from build123d import *

# Parameters (mm, degrees)
SALIENTE_EXTRUIR1_DEPTH = 1.5
CROQUIS2_R              = 1.6
CORTAR_EXTRUIR1_DEPTH   = 10
CROQUIS3_W              = 12
CROQUIS3_H              = 6
CORTAR_EXTRUIR2_DEPTH   = 10
CROQUIS4_W              = 4
CROQUIS4_H              = 16
CORTAR_EXTRUIR3_DEPTH   = 10
CORTAR_EXTRUIR4_REACH   = 107.991
CROQUIS5_R              = 1.5


with BuildPart() as part:
    # Croquis1 → Saliente-Extruir1 (new, symmetric)
    with BuildSketch(Plane.XY):
        Polygon((-75, -32), (-75, -35), (-45, -35), (-45, -32), (45, -32), (45, -35), (75, -35), (75, -32), (97, -32), (97, -12.5), (100, -12.5), (100, 12.5), (97, 12.5), (97, 32), (75, 32), (75, 35), (45, 35), (45, 32), (-45, 32), (-45, 35), (-75, 35), (-75, 32), (-97, 32), (-97, 12.5), (-100, 12.5), (-100, -12.5), (-97, -12.5), (-97, -32), align=None)
    extrude(amount=SALIENTE_EXTRUIR1_DEPTH, both=True)

    # Croquis2 → Cortar-Extruir1 (cut)
    with BuildSketch(Plane.XY.offset(1.5)):
        with Locations((72.948592978, -19.354512833)):
            Circle(CROQUIS2_R)
        with Locations((88.948592978, -19.354512833)):
            Circle(CROQUIS2_R)
    extrude(amount=-CORTAR_EXTRUIR1_DEPTH, mode=Mode.SUBTRACT)

    # Croquis3 → Cortar-Extruir2 (cut)
    with BuildSketch(Plane.XY.offset(1.5)):
        with Locations((81, -25)):
            Rectangle(CROQUIS3_W, CROQUIS3_H)
    extrude(amount=-CORTAR_EXTRUIR2_DEPTH, mode=Mode.SUBTRACT)

    # Croquis4 → Cortar-Extruir3 (cut)
    with BuildSketch(Plane.XY.offset(1.5)):
        with Locations((66.93, 0)):
            Rectangle(CROQUIS4_W, CROQUIS4_H)
    extrude(amount=-CORTAR_EXTRUIR3_DEPTH, mode=Mode.SUBTRACT)

    # Croquis5 → Cortar-Extruir4 (cut, up to next)
    with BuildSketch(Plane.XY.offset(1.5), mode=Mode.PRIVATE) as cortar_extruir4_sk1:
        with Locations((21.93, 9.75)):
            Circle(CROQUIS5_R)
    cortar_extruir4_tool1 = extrude(cortar_extruir4_sk1.sketch, amount=-CORTAR_EXTRUIR4_REACH, mode=Mode.PRIVATE) & part.part
    # Croquis5 → Cortar-Extruir4 (cut, up to next)
    with BuildSketch(Plane.XY.offset(1.5), mode=Mode.PRIVATE) as cortar_extruir4_sk2:
        with Locations((21.93, -9.75)):
            Circle(CROQUIS5_R)
    cortar_extruir4_tool2 = extrude(cortar_extruir4_sk2.sketch, amount=-CORTAR_EXTRUIR4_REACH, mode=Mode.PRIVATE) & part.part
    # Croquis5 → Cortar-Extruir4 (cut, up to next)
    with BuildSketch(Plane.XY.offset(1.5), mode=Mode.PRIVATE) as cortar_extruir4_sk3:
        with Locations((-46.07, -9.75)):
            Circle(CROQUIS5_R)
    cortar_extruir4_tool3 = extrude(cortar_extruir4_sk3.sketch, amount=-CORTAR_EXTRUIR4_REACH, mode=Mode.PRIVATE) & part.part
    # Croquis5 → Cortar-Extruir4 (cut, up to next)
    with BuildSketch(Plane.XY.offset(1.5), mode=Mode.PRIVATE) as cortar_extruir4_sk4:
        with Locations((-46.07, 9.75)):
            Circle(CROQUIS5_R)
    cortar_extruir4_tool4 = extrude(cortar_extruir4_sk4.sketch, amount=-CORTAR_EXTRUIR4_REACH, mode=Mode.PRIVATE) & part.part
    add(cortar_extruir4_tool1.solids().sort_by_distance((21.93, 9.75, 1.5))[0], mode=Mode.SUBTRACT)
    add(cortar_extruir4_tool2.solids().sort_by_distance((21.93, -9.75, 1.5))[0], mode=Mode.SUBTRACT)
    add(cortar_extruir4_tool3.solids().sort_by_distance((-46.07, -9.75, 1.5))[0], mode=Mode.SUBTRACT)
    add(cortar_extruir4_tool4.solids().sort_by_distance((-46.07, 9.75, 1.5))[0], mode=Mode.SUBTRACT)


solid = part.part
Could you check a few things on this model? Use its own coordinates, in mm. Coordinates: 2 decimals unless noted, no trailing zeros. Loops run counter-clockwise (first coordinate to the right, second up) from the corner with the lowest first, then second, coordinate; pieces in that order, holes last. Notation, with made-up numbers: (-29.5, 28.25) -> (-16.5, 28.25) arc R21 cw to (-16.5, 53.25) -> close; hole circle Ø5 at (39.25, 9). An arc over 180 degrees is marked (long way). Answer in a Markdown table with one row per item.
(1) Thinking about a two-plate mould opening in Y: for faces 1 (the face through (87.35, -19.28, 0.02)), 2 (the face through (74.475, -18.874, 0.021)), 3 (the face through (-1, 0, -1.5)), which applies, released by +Y, released by -Y, zero draft, split by the parting line, or undercut?
Results found:
| item | result |
|---|---|
| face 1 | undercut |
| face 2 | undercut |
| face 3 | zero draft |
(2) Imagine slicing it at A-A (y = 15.5). List the corners of the cut face in (x, z) for me, plus the area to 3 significant figures.
Results found:
| item | result |
|---|---|
| outline | (-97, -1.5) -> (97, -1.5) -> (97, 1.5) -> (-97, 1.5) -> close |
| area | 582 mm^2 |
(3) If I drill on probe 1 along Y at (x, z) = (-46.07, -0.9); probe 2 along Y at (x, z) = (21.93, 0.4); probe 3 along X at (y, z) = (-7.5, 0.85), over which ranges is the centre line in solid material (lowest first)?
Results found:
| item | result |
|---|---|
| probe 1 | y = -35 to -11.25, -8.25 to 8.25, 11.25 to 35 |
| probe 2 | y = -32 to -11.25, -8.25 to 8.25, 11.25 to 32 |
| probe 3 | x = -100 to 64.93, 68.93 to 100 |
(4) Will these pins go through, and if not, where does the flat tip stop? pin 1 Ø1.5 at (x, z) = (-98, -0.5) entering from +Y; pin 2 Ø0.9 at (y, z) = (-25.5, 0) entering from -X; pin 3 Ø1.5 at (y, z) = (27, -0.5) entering from +X.
Results found:
| item | result |
|---|---|
| pin 1 | stops at y = 12.5 |
| pin 2 | stops at x = -97 |
| pin 3 | stops at x = 97 |
(5) Imagine slicing it at B-B (z = -0.75). Give the number of separate pieces and of enclosed holes in the cut face, plus the area to 3 significant figures.
Results found:
| item | result |
|---|---|
| separate pieces | 1 |
| enclosed holes | 8 |
| area | 12,700 mm^2 |
